Part model, mm, in its own coordinate system. A direction names the side the tool comes from. Give positions to 0.01 mm unless a question says otherwise; leave off trailing zeros. Loops run counter-clockwise (first coordinate to the right, second up) from the corner with the lowest first, then second, coordinate; pieces in that order, holes last. Notation, with made-up numbers: (23.25, 14) -> (48.25, 14) arc R25 cw to (48.25, 28) -> close; hole circle Ø5 at (21.25, -20). An arc over 180 degrees is marked (long way). One line per question, with ' | ' between items.
Autodesk Inventor part; units mm, degrees
ref_plane "YZ Plane" through (0, 0, 0) normal (1, 0, 0) x (0, 1, 0)
ref_plane "XZ Plane" through (0, 0, 0) normal (0, 1, 0) x (-1, 0, 0)
ref_plane "XY Plane" through (0, 0, 0) normal (0, 0, 1) x (1, 0, 0)
sketch "Sketch1" plane through (0, 0, 0) normal (0, 0, 1) x (1, 0, 0)
  line L0 (0, 35) -> (55, 35)
  line L1 (55, -35) -> (0, -35)
  line L2 (0, -35) -> (0, 35)
  line L3 (11, 12.5) -> (11, -12.5) construction
  circle A0 centre (11, 12.5) radius 11 construction
  circle A1 centre (11, -12.5) radius 11 construction
  circle A2 centre (11, 12.5) radius 4
  circle A3 centre (11, -12.5) radius 4
  line L4 (27.1967, 8.5) -> (37.8033, 8.5) construction
  line L5 (37.8033, 8.5) -> (37.8033, -8.5) construction
  line L6 (37.8033, -8.5) -> (27.1967, -8.5) construction
  line L7 (27.1967, -8.5) -> (27.1967, 8.5) construction
  line L8 (37.8033, 8.5) -> (27.1967, 8.5)
  line L9 (27.1967, 8.5) -> (27.1967, 32.5)
  line L10 (27.1967, 32.5) -> (37.8033, 32.5)
  line L11 (37.8033, 32.5) -> (37.8033, 8.5)
  line L12 (37.8033, -8.5) -> (27.1967, -8.5)
  line L13 (27.1967, -8.5) -> (27.1967, -32.5)
  line L14 (27.1967, -32.5) -> (37.8033, -32.5)
  line L15 (37.8033, -32.5) -> (37.8033, -8.5)
  circle A4 centre (32.5, 8.5) radius 7.5 construction
  line L16 (32.5, 8.5) -> (37.8033, 3.1967) construction
  line L17 (55, 27.8284) -> (45, 27.8284)
  line L18 (45, 27.8284) -> (45, 22.1716)
  line L19 (45, 22.1716) -> (55, 22.1716)
  line L20 (55, -27.8284) -> (45, -27.8284)
  line L21 (45, -27.8284) -> (45, -22.1716)
  line L22 (45, -22.1716) -> (55, -22.1716)
  line L23 (55, -27.8284) -> (55, -35)
  line L24 (55, 35) -> (55, 27.8284)
  line L25 (55, 22.1716) -> (55, -22.1716)
  circle A5 centre (45, 25) radius 4 construction
  line L26 (45, 25) -> (42.1716, 22.1716) construction
  point P0 (0, 0)
  point P1 (0, 0)
  point P2 (11, 0)
  point P3 (27.1967, 0)
  point P4 (45, -25)
  dimension "d7" = 15
  dimension "d16" = 8
  dimension "d0" = 70
  dimension "d2" = 11
  dimension "d3" = 25
  dimension "d4" = 8
  dimension "d5" = 24
  dimension "d6" = 45
  dimension "d9" = 2.5
  dimension "d11" = 22.5
  dimension "d12" = 55
  dimension "d13" = 10
  dimension "d15" = 45
  dimension "d17" = 10
extrude "Extrusion1" add sketch "Sketch1" along normal blind 6.477
sketch "Sketch2" plane through (0, 0, 6.477) normal (0, 0, 1) x (1, 0, 0)
  line L0 (27.1967, 8.5) -> (27.1967, 32.5)
  line L1 (27.1967, 32.5) -> (37.8033, 32.5)
  line L2 (45, 22.1716) -> (45, 27.8284)
  line L3 (45, 27.8284) -> (55, 27.8284)
  line L4 (25, 25.5) -> (40, 25.5) construction
  line L5 (40, 25.5) -> (40, 15.5) construction
  line L6 (40, 15.5) -> (25, 15.5) construction
  line L7 (25, 15.5) -> (25, 25.5) construction
  line L8 (48, 29) -> (52, 29) construction
  line L9 (52, 29) -> (52, 21) construction
  line L10 (52, 21) -> (48, 21) construction
  line L11 (48, 21) -> (48, 29) construction
  line L12 (25, 25.5) -> (23.5, 25.5)
  line L13 (23.5, 25.5) -> (23.5, 29.5)
  line L14 (23.5, 29.5) -> (25, 29.5)
  line L15 (25, 29.5) -> (25, 25.5)
  line L16 (40, 25.5) -> (41.5, 25.5)
  line L17 (41.5, 25.5) -> (41.5, 29.5)
  line L18 (41.5, 29.5) -> (40, 29.5)
  line L19 (40, 29.5) -> (40, 25.5)
  line L20 (40, 15.5) -> (41.5, 15.5)
  line L21 (41.5, 15.5) -> (41.5, 11.5)
  line L22 (41.5, 11.5) -> (40, 11.5)
  line L23 (40, 11.5) -> (40, 15.5)
  line L24 (25, 15.5) -> (23.5, 15.5)
  line L25 (23.5, 15.5) -> (23.5, 11.5)
  line L26 (23.5, 11.5) -> (25, 11.5)
  line L27 (25, 11.5) -> (25, 15.5)
  line L28 (48, 21) -> (52, 21)
  line L29 (52, 21) -> (52, 19.5)
  line L30 (52, 19.5) -> (48, 19.5)
  line L31 (48, 19.5) -> (48, 21)
  line L32 (52, 29) -> (48, 29)
  line L33 (48, 29) -> (48, 30.5)
  line L34 (48, 30.5) -> (52, 30.5)
  line L35 (52, 30.5) -> (52, 29)
  point P0 (0, 0)
  point P1 (25, 20.5)
  point P2 (27.1967, 20.5)
  point P3 (48, 25)
  point P4 (45, 25)
  point P5 (50, 29)
  point P6 (50, 27.8284)
  point P7 (32.5, 25.5)
  point P8 (32.5, 32.5)
  point P9 (25, 27.5)
  dimension "d20" = 4
  dimension "d22" = 1.5
  dimension "d23" = 8
  dimension "d24" = 15
  dimension "d25" = 5
extrude "Extrusion2" cut sketch "Sketch2" against normal through all
mirror "Mirror1" about plane through (0, 0, 0) normal (0, 1, 0) of "Extrusion2"
fillet "Fillet1" radius 5 4 edges at (55, -35, 3.2385) (0, -35, 3.2385) (0, 35, 3.2385) (55, 35, 3.2385)
sketch "Sketch3" plane through (27.1967, 32.5, 0) normal (0, -1, 0) x (1, 0, 0)
  line L0 (10.6066, 0) -> (0, 0)
  line L1 (10.6066, 0) -> (10.6066, 6.477)
  line L2 (0, 6.477) -> (10.6066, 6.477)
  line L3 (0, 0) -> (0, 6.477)
  arc A0 (0, 6.477) -> (10.6066, 6.477) centre (5.3033, 11.7803) ccw
  point P0 (-27.1967, 0)
  dimension "d29" = 15
extrude "Extrusion3" add sketch "Sketch3" along normal up to surface (65 mm away) contours L0 L3 A0 L1
sketch "Sketch4" plane through (45, 22.1716, 0) normal (1, 0, 0) x (0, 0, -1)
  line L0 (0, 5.6569) -> (0, 0)
  line L1 (0, 5.6569) -> (-6.477, 5.6569)
  line L2 (-6.477, 0) -> (-6.477, 5.6569)
  line L3 (0, 0) -> (-6.477, 0)
  arc A0 (-6.477, 0) -> (-6.477, 5.6569) centre (-9.3054, 2.8284) ccw
  point P0 (0, -22.1716)
  dimension "d33" = 8
extrude "Extrusion4" add sketch "Sketch4" along normal up to surface (10 mm away) contours L0 L3 A0 L1
mirror "Mirror2" about plane through (0, 0, 0) normal (0, 1, 0) of "Extrusion4"
properties part number "GANTRY SIDE PLATE"
1) Pull direction Y, two halves, no side cores. Call faces 1 (the flat face through (50, 30.5, 3)), 2 (the flat face through (0, 0, 3)): pulls with the +Y half, pulls with the -Y half, needs draft (parallel to the pull), parting line crosses it, or undercut.
Found:
face 1: undercut | face 2: needs draft
2) Saw through at B-B (y = -12.5). Give the cut face in (x, z), and give its area (3 significant figures).
Found:
outline: (0, 0) -> (7, 0) -> (7, 6.48) -> (0, 6.48) -> close; (15, 0) -> (23.5, 0) -> (23.5, 6.48) -> (15, 6.48) -> close; (25, 0) -> (40, 0) -> (40, 6.48) -> (37.8, 6.48) arc R7.5 cw to (27.2, 6.48) -> (25, 6.48) -> close; (41.5, 0) -> (55, 0) -> (55, 6.48) -> (41.5, 6.48) -> close | area: 269 mm2
3) Saw through at A-A (x = 11). Give the cut face in (y, z), and give its area (3 significant figures).
Found:
outline: (-35, 0) -> (-16.5, 0) -> (-16.5, 6.48) -> (-35, 6.48) -> close; (-8.5, 0) -> (8.5, 0) -> (8.5, 6.48) -> (-8.5, 6.48) -> close; (16.5, 0) -> (35, 0) -> (35, 6.48) -> (16.5, 6.48) -> close | area: 350 mm2
4) Tool access for faces 3 (the flat face through (33, -8.5, 6)), 4 (the flat face through (50, 29, 3)), 5 (the cylindrical face through (49.93, 25.044, 5.306)): list every direction of +Z, -Z, +X, -X, +Y, -Y with a clear straight run to the whole face (end or side of a thin tool).
Found:
face 3: +Z | face 4: +Z, -Z | face 5: +Z, +X
5) Drill centre lines: line 1 (Y direction, x = 11, z = 3); line 2 (Y direction, x = 48.5, z = 1); line 3 (X direction, y = 13.5, z = 2.5). Where is each one in solid material? Low to high.
Found:
line 1: -35 to -16.5, -8.5 to 8.5, 16.5 to 35 | line 2: -35 to -30.5, -29 to -21, -19.5 to 19.5, 21 to 29, 30.5 to 35 | line 3: 0 to 7.13, 14.87 to 23.5, 25 to 40, 41.5 to 55
6) Saw through at C-C (x = 29). Give the cut face in (y, z), and give its area (3 significant figures).
Found:
outline: (-35, 0) -> (35, 0) -> (35, 6.48) -> (32.5, 6.48) -> (32.5, 5.15) -> (8.5, 5.15) -> (8.5, 6.48) -> (-8.5, 6.48) -> (-8.5, 5.15) -> (-32.5, 5.15) -> (-32.5, 6.48) -> (-35, 6.48) -> close | area: 390 mm2
